For this review, use the dimensioned drawing (mm, ordinates from the lowest corner) and the shaded views. Give positions to 0.01 mm unless a question says otherwise; leave off trailing zeros. Order: outer loops, then holes, each group sorted by start corner. A loop starts at its lowest first (then second) coordinate and runs counter-clockwise, first axis right, second up. Notation, with made-up numbers: M 28,-37 L 32,-37 A20 cw 32,-24 Z; hole C 63.5,-16 d3. An arc over 180 degrees is marked long. Answer as CSV lines item,"result". Start each with the question number.
1. For line 1 along Y through (x, z) = (24, 0.75); line 2 along Z through (x, y) = (31, 14); line 3 along X through (y, z) = (40, 44.5), list the stretches that pass through material, from the lowest coordinate up.
2. We need section D-D, the plane z = 12.5. Give the boundary of the cut face in (x, y).
3. Mouldability with a two-part tool opening along Z and no side actions: class the marked faces 1, 2 and 3 as pulls with the +Z half, pulls with the -Z half, needs draft (parallel to the pull), parting line crosses it, or undercut.
4. Clearance check with flat-ended pins moving along their axes: P1, Ø0.6, axis at x = 45.5, z = 1, coming from the -Y side; P2, Ø2, axis at y = 37, z = 1, coming from the +X side; P3, Ø1.5, axis at y = 27, z = 17.5, coming from the +X side (1 decimal). State where each tip first meets the part, or that it passes through.
5. We need section C-C, the plane z = 45. Give the boundary of the cut face in (x, y).
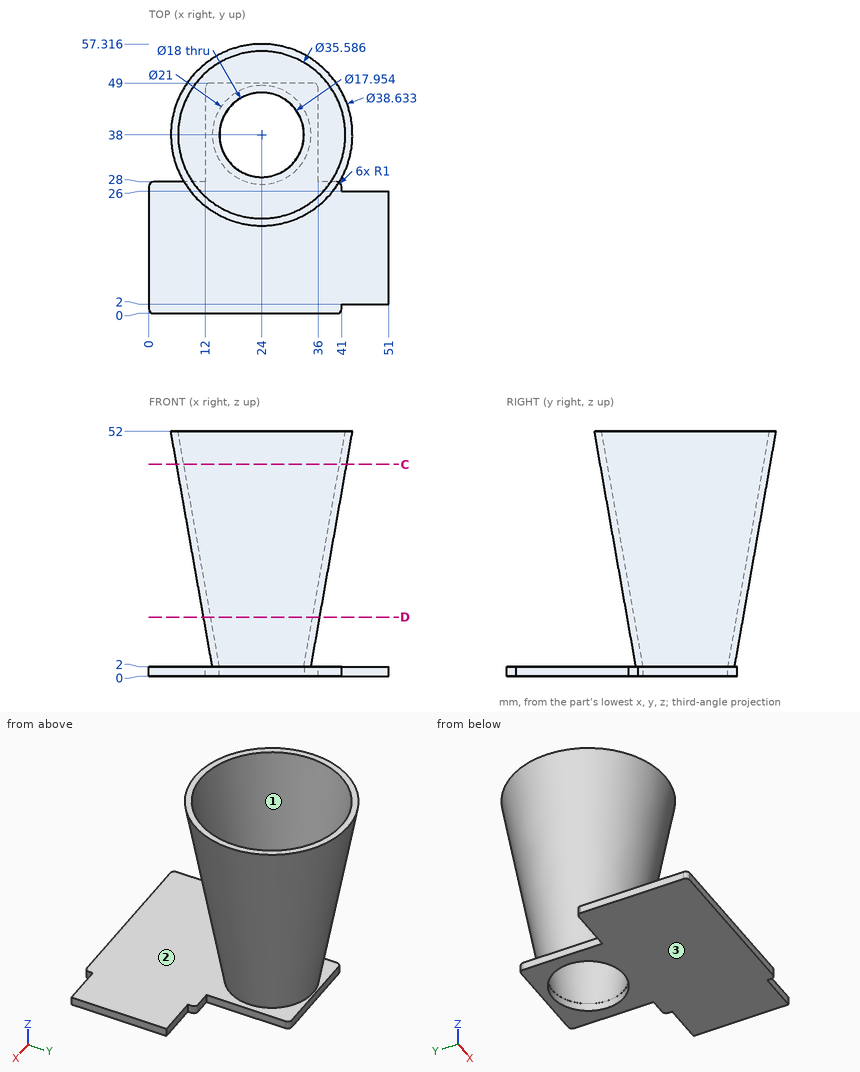
Result set:
1,line 1,"0 to 29, 47 to 49"
1,line 2,"0 to 2"
1,line 3,"6.12 to 7.65, 40.35 to 41.88"
2,outline,"C 24,38 d24.7; hole C 24,38 d21.66"
3,face 1,"pulls with the +Z half"
3,face 2,"undercut"
3,face 3,"pulls with the -Z half"
4,P1,"y = 2"
4,P2,"x = 36"
4,P3,"x = 32.4"
5,outline,"C 24,38 d36.16; hole C 24,38 d33.12"
